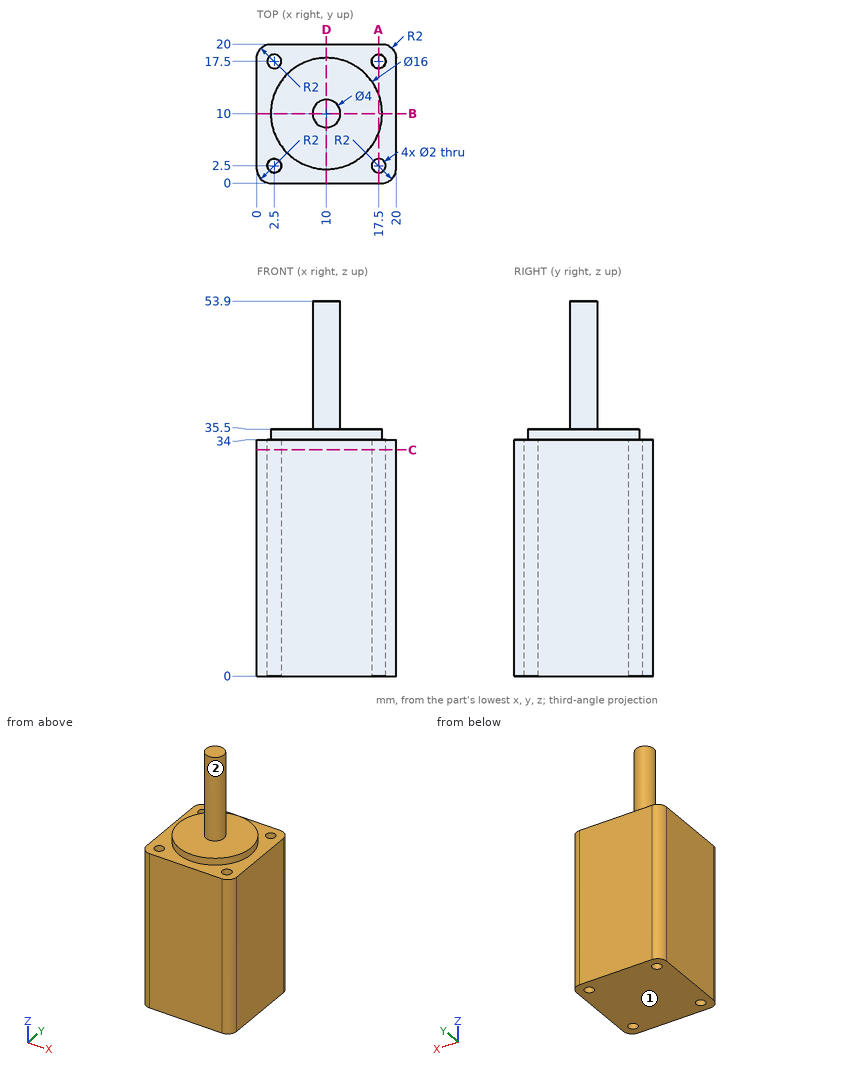
Print and shaded views of the part. All mm, measured from the part's lowest x, y and z. A direction names the side the tool comes from. Give positions to 0.01 mm unless a question says otherwise; leave off trailing zeros. Loops run counter-clockwise (first coordinate to the right, second up) from the corner with the lowest first, then second, coordinate; pieces in that order, holes last.
1) Flat gauge pins, fed straight in: pin 1 Ø1.8 at (x, y) = (2.5, 2.5) entering from +Z; pin 2 Ø5 at (y, z) = (13, 48) entering from -X; pin 3 Ø2 at (x, y) = (15, 3.5) entering from +Z; pin 4 Ø2.5 at (x, y) = (17.5, 2.5) entering from +Z. Where does each tip first touch, or does it go through?
2) Tool access for the marked faces 1 and 2: list every direction of +Z, -Z, +X, -X, +Y, -Y with a clear straight run to the whole face (end or side of a thin tool).
3) Wall check: line 1 (Y direction, x = 17.5, z = 14); line 2 (Y direction, x = 18.25, z = 21.5). Give the ranges that are in metal, low to high.
4) Saw through at B-B (y = 10). Write the cut outline in (x, z).
5) Saw through at A-A (x = 17.5). Write the cut outline in (y, z), plus the area to 3 significant figures.
6) Saw through at C-C (z = 32.5). Write the cut outline in (x, y), plus the area to 3 significant figures.
Answer block:
1. pin 1: passes through
1. pin 2: stops at x = 8.06
1. pin 3: stops at z = 35.5
1. pin 4: stops at z = 34
2. face 1: -Z, +X, -X, +Y, -Y
2. face 2: +Z
3. line 1: y = 0 to 1.5, 3.5 to 16.5, 18.5 to 20
3. line 2: y = 0.02 to 1.84, 3.16 to 16.84, 18.16 to 19.98
4. outline: (0, 0) - (20, 0) - (20, 34) - (18, 34) - (18, 35.5) - (12, 35.5) - (12, 53.9) - (8, 53.9) - (8, 35.5) - (2, 35.5) - (2, 34) - (0, 34) - close
5. outline: (0, 0) - (1.5, 0) - (1.5, 34) - (0, 34) - close; (3.5, 0) - (16.5, 0) - (16.5, 34) - (12.78, 34) - (12.78, 35.5) - (7.22, 35.5) - (7.22, 34) - (3.5, 34) - close; (18.5, 0) - (20, 0) - (20, 34) - (18.5, 34) - close
5. area: 552 mm2
6. outline: (0, 2) arc R2 ccw to (2, 0) - (18, 0) arc R2 ccw to (20, 2) - (20, 18) arc R2 ccw to (18, 20) - (2, 20) arc R2 ccw to (0, 18) - close; hole circle Ø2 at (2.5, 2.5); hole circle Ø2 at (2.5, 17.5); hole circle Ø2 at (17.5, 2.5); hole circle Ø2 at (17.5, 17.5)
6. area: 384 mm2
